Geometry check sheet. Reference: drawing and pictorial views, mm from the part's lowest x, y, z. Give positions to 0.01 mm unless a question says otherwise; leave off trailing zeros. Order: outer loops, then holes, each group sorted by start corner. A loop starts at its lowest first (then second) coordinate and runs counter-clockwise, first axis right, second up. Notation, with made-up numbers: (6, -29.5) -> (30, -29.5) arc R24 cw to (30, 8.5) -> close; hole circle Ø10 at (71.5, 22). An arc over 180 degrees is marked (long way). Write each question's results on one line, items separated by ' | '.
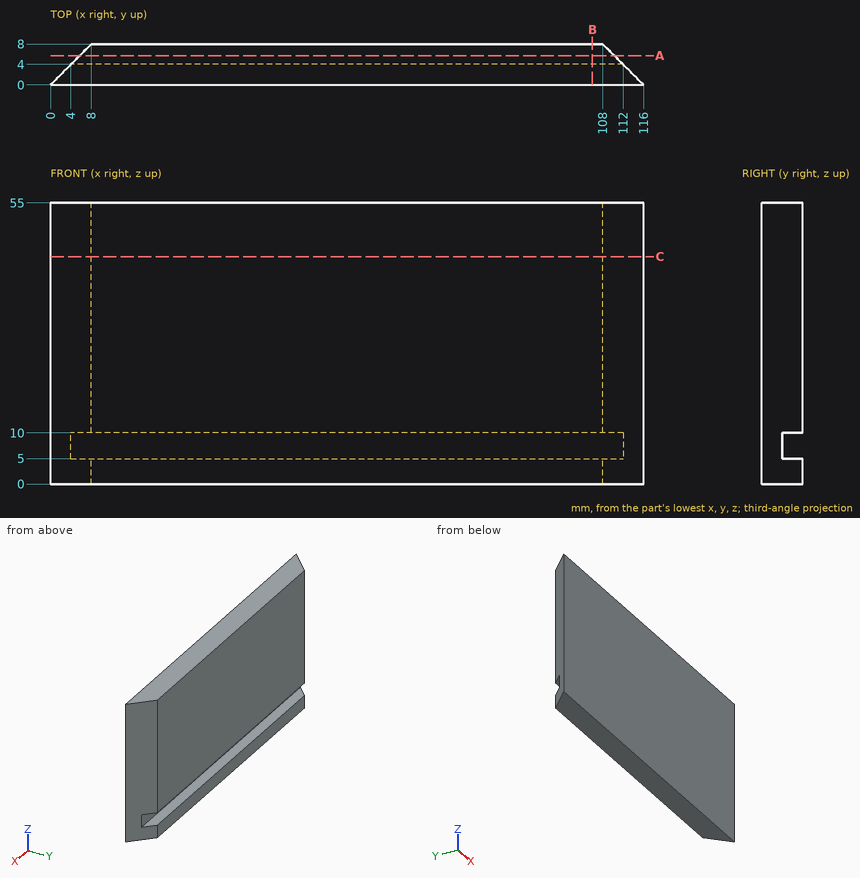
1. Material ranges on probe 1 along Z at (x, y) = (69, 5.75); probe 2 along X at (y, z) = (4, 51.5); probe 3 along X at (y, z) = (1.5, 24), recorded low to high. Write a range as from..to.
Verdict:
probe 1: z = 0..5, 10..55 | probe 2: x = 4..112 | probe 3: x = 1.5..114.5
2. Section check B-B on x = 106. Record the cut outline in (y, z), then the cut area to 3 significant figures.
Verdict:
outline: (0, 0) -> (8, 0) -> (8, 5) -> (4, 5) -> (4, 10) -> (8, 10) -> (8, 55) -> (0, 55) -> close | area: 420 mm^2
3. Section check A-A on y = 5.75. Record the cut outline in (x, z), then the cut area to 4 significant figures.
Verdict:
outline: (5.75, 0) -> (110.25, 0) -> (110.25, 5) -> (5.75, 5) -> close; (5.75, 10) -> (110.25, 10) -> (110.25, 55) -> (5.75, 55) -> close | area: 5,225 mm^2
4. Gauge pin test, flat ends, axial feed: pin 1 Ø4 at (y, z) = (5.5, 37) entering from +X; pin 2 Ø2.5 at (x, z) = (37, 8.5) entering from +Y. Record the tip position at first contact, or that the pin passes through.
Verdict:
pin 1: stops at x = 112.5 | pin 2: stops at y = 4
5. Section check C-C on z = 44.5. Record the cut outline in (x, y).
Verdict:
outline: (0, 0) -> (116, 0) -> (108, 8) -> (8, 8) -> close
